The listing builds one solid part. Answer for the finished solid, in the listing's coordinates (mm). A direction names the side the tool comes from. Coordinates: 2 decimals unless noted, no trailing zeros. Loops run counter-clockwise (first coordinate to the right, second up) from the corner with the lowest first, then second, coordinate; pieces in that order, holes last. Notation, with made-up numbers: (-18.5, 34.25) - (1.5, 34.25) arc R18 cw to (1.5, 48.25) - close; hole circle Ø7 at (31.5, 77). An arc over 180 degrees is marked (long way). Put each result on its own line as item: value.
Solid Edge part; units mm, degrees
sketch "Sketch1" plane through (0, 0, 0) normal (-1, 0, 0) x (0, -1, 0)
  line L0 (25, -17.5) -> (25, 17.5)
  line L1 (25, 17.5) -> (-25, 17.5)
  line L2 (-25, 17.5) -> (-25, -17.5)
  line L3 (-25, -17.5) -> (25, -17.5)
extrude "Protrusion1" add sketch "Sketch1" along normal blind 100
sketch "Sketch2" plane through (-50, 0, 17.5) normal (0, 0, 1) x (0, 1, 0)
  line L0 (20, 45) -> (20, -45)
  line L1 (-20, -45) -> (20, -45)
  line L2 (-20, 45) -> (-20, -45)
  line L3 (-20, 45) -> (20, 45)
extrude "Cutout1" cut sketch "Sketch2" against normal blind 30
sketch "Sketch3" plane through (-5, 0, 2.5) normal (-1, 0, 0) x (0, 1, 0)
  line L0 (-20, 15) -> (20, 15)
  line L1 (20, 15) -> (20, -15)
  line L2 (20, -15) -> (-20, -15)
  line L3 (-20, -15) -> (-20, 15)
  line L4 (11.5947, -3.85) -> (8.4053, -3.85)
  line L5 (8.4053, -3.85) -> (6.15, -1.5947)
  line L6 (6.15, -1.5947) -> (6.15, 1.5947)
  line L7 (6.15, 1.5947) -> (8.4053, 3.85)
  line L8 (8.4053, 3.85) -> (11.5947, 3.85)
  line L9 (11.5947, 3.85) -> (13.85, 1.5947)
  line L10 (13.85, 1.5947) -> (13.85, -1.5947)
  line L11 (13.85, -1.5947) -> (11.5947, -3.85)
  line L12 (-11.5947, -3.85) -> (-8.4053, -3.85)
  line L13 (-8.4053, -3.85) -> (-6.15, -1.5947)
  line L14 (-6.15, -1.5947) -> (-6.15, 1.5947)
  line L15 (-6.15, 1.5947) -> (-8.4053, 3.85)
  line L16 (-8.4053, 3.85) -> (-11.5947, 3.85)
  line L17 (-11.5947, 3.85) -> (-13.85, 1.5947)
  line L18 (-13.85, 1.5947) -> (-13.85, -1.5947)
  line L19 (-13.85, -1.5947) -> (-11.5947, -3.85)
extrude "Protrusion2" add sketch "Sketch3" along normal blind 5
sketch "Sketch4" plane through (0, 0, 0) normal (1, 0, 0) x (0, 1, 0)
  circle A0 centre (-10, 2.5) radius 2.5
  circle A1 centre (10, 2.5) radius 2.5
extrude "ExtrudedProtrusion_27" add sketch "Sketch4" along normal blind 5
chamfer "Chamfer_14" distance 2 angle 45 2 edges at (0, 7.5, 2.5) (0, -12.5, 2.5)
sketch "Sketch5" plane through (-100, 0, 0) normal (-1, 0, 0) x (0, -1, 0)
  circle A0 centre (-10, 2.5) radius 2.5
  circle A1 centre (10, 2.5) radius 2.5
extrude "ExtrudedProtrusion_29" add sketch "Sketch5" along normal blind 5
sketch "Sketch6" plane through (-105, 10, 2.5) normal (-1, 0, 0) x (0, -1, 0)
  circle A0 centre (0, 0) radius 2.5
  circle A1 centre (20, 0) radius 2.5
extrude "ExtrudedCutout_41" cut sketch "Sketch6" against normal blind 159
sketch "Sketch7" plane through (-95, 0, 2.5) normal (1, 0, 0) x (0, -1, 0)
  line L0 (-20, 15) -> (20, 15)
  line L1 (20, 15) -> (20, -15)
  line L2 (20, -15) -> (-20, -15)
  line L3 (-20, -15) -> (-20, 15)
  line L4 (-11.5947, 3.85) -> (-8.4053, 3.85)
  line L5 (-8.4053, 3.85) -> (-6.15, 1.5947)
  line L6 (-6.15, 1.5947) -> (-6.15, -1.5947)
  line L7 (-6.15, -1.5947) -> (-8.4053, -3.85)
  line L8 (-8.4053, -3.85) -> (-11.5947, -3.85)
  line L9 (-11.5947, -3.85) -> (-13.85, -1.5947)
  line L10 (-13.85, -1.5947) -> (-13.85, 1.5947)
  line L11 (-13.85, 1.5947) -> (-11.5947, 3.85)
  line L12 (6.15, 1.5947) -> (6.15, -1.5947)
  line L13 (6.15, -1.5947) -> (8.4053, -3.85)
  line L14 (8.4053, -3.85) -> (11.5947, -3.85)
  line L15 (11.5947, -3.85) -> (13.85, -1.5947)
  line L16 (13.85, -1.5947) -> (13.85, 1.5947)
  line L17 (13.85, 1.5947) -> (11.5947, 3.85)
  line L18 (11.5947, 3.85) -> (8.4053, 3.85)
  line L19 (8.4053, 3.85) -> (6.15, 1.5947)
extrude "ExtrudedProtrusion_30" add sketch "Sketch7" along normal blind 5
sketch "Sketch8" plane through (0, 0, 0) normal (1, 0, 0) x (0, -1, 0)
  line L0 (-25, 11.5) -> (-21.85, 11.5)
  line L1 (-21.85, 11.5) -> (-21.85, 14.65)
  line L2 (-21.85, 14.65) -> (-25, 14.65)
  line L3 (-25, 14.65) -> (-21.85, 17.5)
  line L4 (-21.85, 17.5) -> (-21.85, 20.916)
  line L5 (-21.85, 20.916) -> (-29.169, 20.916)
  line L6 (-29.169, 20.916) -> (-29.169, 11.5)
  line L7 (-29.169, 11.5) -> (-25, 11.5)
extrude "Cutout2" cut sketch "Sketch8" against normal blind 112
fillet "Round_8" radius 2 1 edges at (-50, -25, -17.5)
chamfer "Chamfer_17" distance 2 angle 45 2 edges at (-100, -10, 0) (-100, 10, 0)
sketch "Sketch9" plane through (-100, 0, 0) normal (-1, 0, 0) x (0, 1, 0)
  line L0 (-22, -17.5) -> (-22, -14.5)
  line L1 (-22, -14.5) -> (-19, -14.5)
  line L2 (-19, -14.5) -> (-19, -20.07)
  line L3 (-27.2533, -20.0192) -> (-19, -20.07)
  line L4 (-27.2533, -14.5) -> (-27.2533, -20.0192)
  line L5 (-25, -14.5) -> (-27.2533, -14.5)
  line L6 (-25, -14.5) -> (-22, -17.5)
extrude "ExtrudedCutout_43" cut sketch "Sketch9" against normal blind 234
1) The part is cut by section A-A (y = -10). Give the vertices of the cut face in (x, z), and give its area (3 significant figures).
Found:
outline: (-100, -17.5) - (0, -17.5) - (0, -2) - (2, 0) - (-5, 0) - (-5, -1.35) - (-10, -1.35) - (-10, -12.5) - (-90, -12.5) - (-90, -1.35) - (-95, -1.35) - (-95, 0) - (-98, 0) - (-100, -2) - close; (-100, 7) - (-98, 5) - (-95, 5) - (-95, 6.35) - (-90, 6.35) - (-90, 17.5) - (-100, 17.5) - close; (-10, 6.35) - (-5, 6.35) - (-5, 5) - (2, 5) - (0, 7) - (0, 17.5) - (-10, 17.5) - close
area: 973 mm^2
2) Straight lines are drawn through the part: L1, parallel to X at y = 7.5, z = -8; L2, parallel to Y at x = -51.5, z = 1; L3, parallel to Z at x = -2.75, y = 10. For each, find the intervals that lie inside material, in ascending order. Write a range as [from, to].
Found:
L1: x = [-100, -90], [-10, 0]
L2: y = [-25, -20], [20, 25]
L3: z = [-17.5, 0], [5, 17.5]
3) For a pull along Z with two mould halves and no side action, classify faces 4 (the face through (-7, 10, 6.35)), 5 (the face through (-49.3, 23.4, -16.1)), 6 (the face through (0, 0, 0)), 7 (the face through (-98.125, 7.496, 3.289)) as pulls with the +Z half, pulls with the -Z half, needs draft (parallel to the pull), parting line crosses it, or undercut.
Found:
face 4: undercut
face 5: pulls with the -Z half
face 6: needs draft
face 7: undercut
4) The part is cut by section D-D (y = 16). Give the vertices of the cut face in (x, z).
Found:
outline: (-100, -17.5) - (0, -17.5) - (0, 17.5) - (-10, 17.5) - (-10, -12.5) - (-90, -12.5) - (-90, 17.5) - (-100, 17.5) - close
5) The part is cut by section B-B (z = -6.5). Give the vertices of the cut face in (x, y).
Found:
outline: (-100, -25) - (0, -25) - (0, 25) - (-100, 25) - close; hole (-90, -20) - (-10, -20) - (-10, 20) - (-90, 20) - close
6) For faces 1 (the face through (-95, -19, 16)), 2 (the face through (-49, -25, -1)), 3 (the face through (-92.535, -7.262, 5.207)), determine the directions among +Z, -Z, +X, -X, +Y, -Y from which every point of the face is accessible in a straight line to the end or side of a thin tool.
Found:
face 1: +Z, +X, -X
face 2: +Z, -Z, +X, -X, -Y
face 3: none
7) The part is cut by section C-C (x = -6.5). State how many separate pieces and enclosed holes the cut face has, and give its area (3 significant figures).
Found:
separate pieces: 1
enclosed holes: 2
area: 1,620 mm^2
8) Each of these flat-tipped pins is pushed along its axis until it touches: pin 1 (1 mm diameter, centred on x = -18, y = 6.5, fed in from +Z); pin 2 (1.5 mm diameter, centred on x = -95, z = 15.5, fed in from -Y); pin 3 (0.9 mm diameter, centred on x = -67.5, z = -13.5, fed in from +Y). Where does it stop, or does it pass through?
Found:
pin 1: stops at z = -12.5
pin 2: stops at y = -24.75
pin 3: stops at y = 21.85
